CAD build for the part. Positions are in the model's coordinates, mm. A direction names the side the tool comes from. Give positions to 0.01 mm unless a question says otherwise; leave off trailing zeros. Order: outer loops, then holes, each group sorted by start corner. A loop starts at its lowest first (then second) coordinate and runs counter-clockwise, first axis right, second up. Notation, with made-up numbers: (76, 8.25) -> (90, 8.25) arc R17 ccw to (90, 30.25) -> close; hole circle Ø2 at (80, 38). An arc over 180 degrees is marked (long way). Use one line per item in the form item = value. Start each with the question number.
1) Cut at B-B, the plane z = 0. Give the cut face in (x, y), and give its area (3 significant figures).
2) Cut at A-A, the plane x = 0. Give the cut face in (y, z) (3 decimals), and give its area (3 significant figures).
3) Probe line 1 (Z direction, x = 0.5, y = 4.7); line 2 (Z direction, x = -31, y = 2); line 3 (Z direction, x = -1.5, y = 0.55). List the from-to ranges inside material, lowest first.
4) Tool access for faces 4 (the face through (29.88, 2.5, 18.44)), 5 (the face through (5.08, 3, -35)), 6 (the face through (-24.58, 2.5, 11.89)): list every direction of +Z, -Z, +X, -X, +Y, -Y with a clear straight run to the whole face (end or side of a thin tool).
5) Cut at D-D, the plane x = 12. Give the cut face in (y, z).
6) Drop flat-ended pins along their axis: P1, Ø4, axis at x = -19.89, z = 23.71, coming from the -Y side; P2, Ø1, axis at x = 18.5, y = 3.5, coming from the +Z side; P3, Ø3, axis at y = 0.5, z = -23.5, coming from the -X side; P4, Ø1.5, axis at y = 4, z = -33.5, coming from the +X side. Give the stop position or say it passes through.
7) Mould opens along X. For faces 1 (the face through (16, 5.08, -13)), 2 (the face through (24.856, 2.504, 13.266)), 3 (the face through (29.3, 2.5, 23.05)) say: pulls with the +X half, pulls with the -X half, needs draft (parallel to the pull), parting line crosses it, or undercut.
8) Cut at C-C, the plane z = -38. Give the cut face in (x, y), and give its area (3 significant figures).
from build123d import *

# Parameters (mm, degrees)
SKETCH1_R               = 20.32
SKETCH1_R_2             = 3.3274
BOSS_EXTRUDE1_DEPTH     = 5.08
F_1_4_20_TAPPED_HOLE1_D = 5.1054


with BuildPart() as part:
    # Sketch1 → Boss-Extrude1 (new body)
    with BuildSketch(Plane(origin=(0, 0, 0), x_dir=(1, 0, 0), z_dir=(0, 1, 0))):
        with BuildLine():
            Line((19.57652647, -23.05812517), (27.015058429, -29.299794594))
            ThreePointArc((27.015058429, -29.299794594), (34.171925257, -28.67364988), (33.545780543, -21.516783052))
            Line((33.545780543, -21.516783052), (26.107248584, -15.275113628))
            ThreePointArc((26.107248584, -15.275113628), (24.848469725, -13.233023939), (25.059583331, -10.843445406))
            ThreePointArc((25.059583331, -10.843445406), (25.400007253, -10.020112603), (25.713388999, -9.186111864))
            ThreePointArc((25.713388999, -9.186111864), (27.657978886, -6.682698723), (30.708135247, -5.81953399))
            ThreePointArc((30.708135247, -5.81953399), (36.774453721, 0), (30.708135247, 5.81953399))
            ThreePointArc((30.708135247, 5.81953399), (27.657978886, 6.682698723), (25.713388999, 9.186111864))
            ThreePointArc((25.713388999, 9.186111864), (24.562302912, 11.927124576), (23.12004719, 14.526749221))
            ThreePointArc((23.12004719, 14.526749221), (22.572337736, 17.077966647), (23.794690624, 19.383297298))
            ThreePointArc((23.794690624, 19.383297298), (23.638163205, 28.170865922), (14.956916793, 26.79907006))
            ThreePointArc((14.956916793, 26.79907006), (12.898868646, 25.194970992), (10.291301197, 25.291345252))
            ThreePointArc((10.291301197, 25.291345252), (9.056948556, 25.759167453), (7.801428571, 26.166786911))
            ThreePointArc((7.801428571, 26.166786911), (5.835204005, 27.541055979), (5.08, 29.81796648))
            Line((5.08, 29.81796648), (5.08, 39.528280321))
            ThreePointArc((5.08, 39.528280321), (0, 44.608280321), (-5.08, 39.528280321))
            Line((-5.08, 39.528280321), (-5.08, 29.81796648))
            ThreePointArc((-5.08, 29.81796648), (-5.835204005, 27.541055979), (-7.801428571, 26.166786911))
            ThreePointArc((-7.801428571, 26.166786911), (-18.785541793, 19.815812992), (-25.713388999, 9.186111864))
            ThreePointArc((-25.713388999, 9.186111864), (-27.657978886, 6.682698723), (-30.708135247, 5.81953399))
            ThreePointArc((-30.708135247, 5.81953399), (-36.774453721, 0), (-30.708135247, -5.81953399))
            ThreePointArc((-30.708135247, -5.81953399), (-27.657978886, -6.682698723), (-25.713388999, -9.186111864))
            ThreePointArc((-25.713388999, -9.186111864), (-24.562302912, -11.927124576), (-23.12004719, -14.526749221))
            ThreePointArc((-23.12004719, -14.526749221), (-22.572337736, -17.077966647), (-23.794690624, -19.383297298))
            ThreePointArc((-23.794690624, -19.383297298), (-23.638163205, -28.170865922), (-14.956916793, -26.79907006))
            ThreePointArc((-14.956916793, -26.79907006), (-12.898868646, -25.194970992), (-10.291301197, -25.291345252))
            ThreePointArc((-10.291301197, -25.291345252), (2.67791157, -27.173365905), (15.030260084, -22.795927417))
            ThreePointArc((15.030260084, -22.795927417), (17.346876056, -22.173075144), (19.57652647, -23.05812517))
        make_face()
        Circle(SKETCH1_R, mode=Mode.SUBTRACT)
        with Locations((-30.9499, 0)):
            Circle(SKETCH1_R_2, mode=Mode.SUBTRACT)
        with Locations((30.9499, 0)):
            Circle(SKETCH1_R_2, mode=Mode.SUBTRACT)
    extrude(amount=BOSS_EXTRUDE1_DEPTH)

    # 1/4-20 Tapped Hole1 (through all)
    with Locations(Plane(origin=(0, 5.08, -39.528280321), x_dir=(0, 0, 1), z_dir=(0, 1, 0))):
        with Locations((0, 0), (15.819281411, 19.894212241), (64.936569144, 30.280419486), (63.237279231, -19.894212241)):
            Hole(F_1_4_20_TAPPED_HOLE1_D / 2)


solid = part.part
Result:
q1.outline = (-36.77, 0) -> (-34.28, 0) -> (-34.28, 5.08) -> (-36.77, 5.08) -> close; (-27.62, 0) -> (-20.32, 0) -> (-20.32, 5.08) -> (-27.62, 5.08) -> close; (20.32, 0) -> (27.62, 0) -> (27.62, 5.08) -> (20.32, 5.08) -> close; (34.28, 0) -> (36.77, 0) -> (36.77, 5.08) -> (34.28, 5.08) -> close
q1.area = 99.6 mm²
q2.outline = (0, -44.608) -> (5.08, -44.608) -> (5.08, -42.081) -> (0, -42.081) -> close; (0, -36.976) -> (5.08, -36.976) -> (5.08, -20.32) -> (0, -20.32) -> close; (0, 20.32) -> (5.08, 20.32) -> (5.08, 27.305) -> (0, 27.305) -> close
q2.area = 133 mm²
q3.line_1 = -44.58 to -42.03, -37.03 to -20.31, 20.31 to 27.3
q3.line_2 = -5.82 to -3.33, 3.33 to 5.82
q3.line_3 = -44.38 to -41.59, -37.46 to -20.26, 20.26 to 27.26
q4.face_4 = +X, +Y, -Y
q4.face_5 = -Z, +X, +Y, -Y
q4.face_6 = -X, +Y, -Y
q5.outline = (0, -25.02) -> (5.08, -25.02) -> (5.08, -16.4) -> (0, -16.4) -> close; (0, 16.4) -> (5.08, 16.4) -> (5.08, 24.53) -> (0, 24.53) -> close
q6.P1 = through
q6.P2 = 22.66
q6.P3 = -16.17
q6.P4 = 5.08
q7.face_1 = needs draft
q7.face_2 = pulls with the +X half
q7.face_3 = undercut
q8.outline = (-5.08, 0) -> (-2.04, 0) -> (-2.04, 5.08) -> (-5.08, 5.08) -> close; (2.04, 0) -> (5.08, 0) -> (5.08, 5.08) -> (2.04, 5.08) -> close
q8.area = 30.8 mm²
